Source: CAD feature listing. Evaluate the final solid. Frame: model axes, mm. Face numbers are marked on the shaded views. A direction names the side the tool comes from. Coordinates: 2 decimals unless noted, no trailing zeros. Loops run counter-clockwise (first coordinate to the right, second up) from the corner with the lowest first, then second, coordinate; pieces in that order, holes last.
Item 1: Section query A-A, the plane z = 0. Return the cut outline in (x, y), then the cut area to 3 significant figures.
Item 2: Reachability of the marked faces 1 and 2 from +Z, -Z, +X, -X, +Y, -Y: full face, straight path, thin tool, end or side. Return the list, or none.
Item 3: Line query: probe 1 along X at (y, z) = (1.15, 0); probe 2 along Y at (x, z) = (-2, -6.5); probe 3 along Z at (x, y) = (1.25, 0.55). Output: solid intervals per line, ascending.
Item 4: Section query C-C, the plane y = 0.5. Return the cut outline in (x, z).
Item 5: Pull-direction query (X, two-part tool) for the marked faces 3, 4 and 5; classes: +X half, -X half, draft (parallel to the pull), parting line (faces both ways), or undercut.
Item 6: Section query D-D, the plane y = 3.15. Return the cut outline in (x, z).
Item 7: Pin query (flat end, axial travel): pin 1 Ø1.8 at (x, z) = (0, 7) entering from +Y; pin 2 Ø2 at (y, z) = (1.5, -2.5) entering from -X; pin 3 Ø3.5 at (x, z) = (0, -7) entering from +Y; pin 4 Ø1.8 at (x, z) = (0.5, -0.5) entering from +Y. Return the tip coordinate at first contact, or that it passes through.
Item 8: Section query B-B, the plane x = 0. Return the cut outline in (y, z), then the cut area to 3 significant figures.
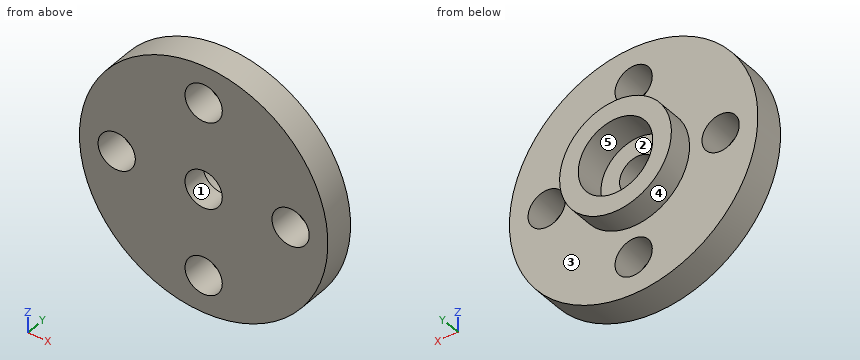
```python
from build123d import *

# Parameters (mm, degrees)
SKETCH_1_R          = 10
SKETCH_1_R_2        = 1.5
EXTRUDE_1_DEPTH     = 2.5
SKETCH_2_R          = 4.5
SKETCH_2_R_2        = 3
EXTRUDE_2_DEPTH     = 2
CUT_EXTRUDE_START   = -0.5
SKETCH_3_R          = 3
CUT_EXTRUDE_1_DEPTH = 0.5


with BuildPart() as part:
    # 草图1 → 凸台-拉伸1 (new body)
    with BuildSketch(Plane(origin=(0, 0, 0), x_dir=(1, 0, 0), z_dir=(0, 1, 0))):
        with Locations(Location((0, 0, 0), (0, 0, 270))):
            Circle(SKETCH_1_R)
        with Locations(Location((0, 0, 0), (0, 0, 270))):
            Circle(SKETCH_1_R_2, mode=Mode.SUBTRACT)
        with Locations(Location((0, 7, 0), (0, 0, 270))):
            Circle(SKETCH_1_R_2, mode=Mode.SUBTRACT)
        with Locations(Location((7, 0, 0), (0, 0, 270))):
            Circle(SKETCH_1_R_2, mode=Mode.SUBTRACT)
        with Locations(Location((0, -7, 0), (0, 0, 270))):
            Circle(SKETCH_1_R_2, mode=Mode.SUBTRACT)
        with Locations(Location((-7, 0, 0), (0, 0, 270))):
            Circle(SKETCH_1_R_2, mode=Mode.SUBTRACT)
    extrude(amount=EXTRUDE_1_DEPTH)

    # 草图2 → 凸台-拉伸2 (add)
    with BuildSketch(Plane(origin=(0, 2.5, 0), x_dir=(1, 0, 0), z_dir=(0, 1, 0))):
        with Locations(Location((0, 0, 0), (0, 0, 270))):
            Circle(SKETCH_2_R)
        with Locations(Location((0, 0, 0), (0, 0, 270))):
            Circle(SKETCH_2_R_2, mode=Mode.SUBTRACT)
    extrude(amount=EXTRUDE_2_DEPTH)

    # 草图3 → 切除-拉伸1 (cut)
    with BuildSketch(Plane(origin=(0, 2.5, 0), x_dir=(1, 0, 0), z_dir=(0, 1, 0)).offset(CUT_EXTRUDE_START)):
        with Locations(Location((0, 0, 0), (0, 0, 270))):
            Circle(SKETCH_3_R)
    extrude(amount=CUT_EXTRUDE_1_DEPTH, mode=Mode.SUBTRACT)


solid = part.part
```
Verdict:
1. outline: (-10, 0) - (-8.5, 0) - (-8.5, 2.5) - (-10, 2.5) - close; (-5.5, 0) - (-1.5, 0) - (-1.5, 2) - (-3, 2) - (-3, 4.5) - (-4.5, 4.5) - (-4.5, 2.5) - (-5.5, 2.5) - close; (1.5, 0) - (5.5, 0) - (5.5, 2.5) - (4.5, 2.5) - (4.5, 4.5) - (3, 4.5) - (3, 2) - (1.5, 2) - close; (8.5, 0) - (10, 0) - (10, 2.5) - (8.5, 2.5) - close
1. area: 32.0 mm2
2. face 1: +Y, -Y
2. face 2: +Y
3. probe 1: x = -10 to -8.5, -5.5 to -1.5, 1.5 to 5.5, 8.5 to 10
3. probe 2: y = 0 to 2.5
3. probe 3: z = -9.92 to -7.83, -6.17 to -0.83, 0.83 to 6.17, 7.83 to 9.92
4. outline: circle Ø20 at (0, 0); hole circle Ø3 at (-7, 0); hole circle Ø3 at (0, -7); hole circle Ø3 at (0, 0); hole circle Ø3 at (0, 7); hole circle Ø3 at (7, 0)
5. face 3: draft
5. face 4: parting line
5. face 5: undercut
6. outline: circle Ø9 at (0, 0); hole circle Ø6 at (0, 0)
7. pin 1: passes through
7. pin 2: stops at x = -9.89
7. pin 3: stops at y = 2.5
7. pin 4: stops at y = 2
8. outline: (0, -10) - (2.5, -10) - (2.5, -8.5) - (0, -8.5) - close; (0, -5.5) - (2.5, -5.5) - (2.5, -4.5) - (4.5, -4.5) - (4.5, -3) - (2, -3) - (2, -1.5) - (0, -1.5) - close; (0, 1.5) - (2, 1.5) - (2, 3) - (4.5, 3) - (4.5, 4.5) - (2.5, 4.5) - (2.5, 5.5) - (0, 5.5) - close; (0, 8.5) - (2.5, 8.5) - (2.5, 10) - (0, 10) - close
8. area: 32.0 mm2
